Build history of the part. All positions in model axes, mm. A direction names the side the tool comes from. Give positions to 0.01 mm unless a question says otherwise; leave off trailing zeros. Write each loop counter-clockwise with the first axis right and the second up, starting at its lowest first coordinate (ties: lowest second). Pieces come first, ordered by that corner, then holes. Notation, with made-up numbers: (53.5, 31.25) -> (59.5, 31.25) arc R6 ccw to (59.5, 38.25) -> close; hole circle Ø5 at (-24, 19.5). An arc over 180 degrees is marked (long way). Write item = value, one per line. Start each with the question number.
Q1. Saw through at B-B, the plane y = 11. List the corners of the cut face in (x, z).
Q2. Drop flat-ended pins along their axis: P1, Ø3.5, axis at x = 8.5, z = -33, coming from the +Y side; P2, Ø8, axis at y = 14.5, z = 23.5, coming from the -X side; P3, Ø2.5, axis at x = 2.5, y = 2, coming from the +Z side. Give the stop position or say it passes through.
Q3. Saw through at D-D, the plane x = -16. List the corners of the cut face in (y, z), then the cut area to 3 significant figures.
Q4. Wall check: line 1 (Z direction, x = 33.5, y = 1.2); line 2 (Z direction, x = -30.5, y = 1.1); line 3 (Z direction, x = -2, y = 9.5). Give the ranges that are in metal, low to high.
Q5. Saw through at C-C, the plane z = 24. List the corners of the cut face in (x, y), then the cut area to 3 significant figures.
Q6. Saw through at A-A, the plane x = 23.5. List the corners of the cut face in (y, z).
Q7. Mould opens along X. For faces 4 (the face through (-37.5, 10, -19)), 5 (the face through (24, 20, 7.5)), 6 (the face through (1, 3, 0)), 7 (the face through (23.175, 32.536, 12.91)) say: pulls with the +X half, pulls with the -X half, needs draft (parallel to the pull), parting line crosses it, or undercut.
Q8. Tool access for faces 1 (the face through (24, 36, 18.171)), 2 (the face through (-9, 1, 31)), 3 (the face through (34.5, 12, -26)): list every direction of +Z, -Z, +X, -X, +Y, -Y with a clear straight run to the whole face (end or side of a thin tool).
Autodesk Inventor part; units mm, degrees
ref_plane "YZ Plane" through (0, 0, 0) normal (1, 0, 0) x (0, 1, 0)
ref_plane "XZ Plane" through (0, 0, 0) normal (0, 1, 0) x (-1, 0, 0)
ref_plane "XY Plane" through (0, 0, 0) normal (0, 0, 1) x (1, 0, 0)
sketch "Sketch1" plane through (0, 0, 0) normal (0, 1, 0) x (-1, 0, 0)
  line L0 (37.5, -31) -> (-37.5, -31)
  line L1 (-37.5, -31) -> (-37.5, 31)
  line L2 (-37.5, 31) -> (37.5, 31)
  line L3 (37.5, 31) -> (37.5, -31)
  line L4 (37.5, -31) -> (-37.5, 31) construction
  line L5 (-37.5, -31) -> (37.5, 31) construction
  point P0 (0, 0)
  dimension "d0" = 75
  dimension "d1" = 62
extrude "Extrusion1" add sketch "Sketch1" along normal blind 3
sketch "Sketch2" plane through (0, 3, 0) normal (0, 1, 0) x (1, 0, 0)
  line L0 (37.5, 31) -> (-37.5, 31)
  line L1 (-37.5, 31) -> (-37.5, -31)
  circle A0 centre (-30.5, -7.5) radius 2.5
  circle A1 centre (-30.5, -20) radius 2.5
  circle A2 centre (-16, 1) radius 2.5
  line L2 (-37.5, -31) -> (37.5, -31)
  line L3 (37.5, -31) -> (37.5, 31)
  line L4 (-30.5, -7.5) -> (-30.5, -31)
  point P0 (0, 0)
  dimension "d4" = 5
  dimension "d5" = 5
  dimension "d6" = 12.5
  dimension "d7" = 7
  dimension "d8" = 5
  dimension "d9" = 8.5
  dimension "d10" = 14.5
  dimension "d11" = 30
extrude "Extrusion2" cut sketch "Sketch2" against normal through all contours A0 | A1 L4 | L4 A1 | A2
sketch "Sketch3" plane through (0, 3, 0) normal (0, 1, 0) x (1, 0, 0)
  line L0 (-37.5, 31) -> (-37.5, -31)
  line L1 (37.5, -31) -> (37.5, 31)
  line L2 (-37.5, -20) -> (37.5, -20)
  line L3 (19.5, -32.5) -> (27.5, -32.5)
  line L4 (27.5, -32.5) -> (27.5, -7.5)
  line L5 (27.5, -7.5) -> (19.5, -7.5)
  line L6 (19.5, -7.5) -> (19.5, -32.5)
  line L7 (19.5, -32.5) -> (27.5, -7.5) construction
  line L8 (27.5, -32.5) -> (19.5, -7.5) construction
  circle A0 centre (-30.5, -20) radius 2.5
  point P0 (0, 0)
  point P1 (23.5, -20)
  dimension "d16" = 8
  dimension "d21" = 25
  dimension "d22" = 0
  dimension "d74" = 50
extrude "Extrusion3" add sketch "Sketch3" along normal blind 35 contours L6 L5 L4 L2 | L2 L4 L3 L6
sketch "Sketch4" plane through (27.5, 3, 32.5) normal (1, 0, 0) x (0, 0, -1)
  line L0 (25, 0) -> (1.5, 0)
  circle A0 centre (12.5, 18.5) radius 9
  line L1 (0, 35) -> (25, 35)
  line L2 (10.6712, 35) -> (14.3288, 35)
  line L3 (14.3288, 35) -> (14.3288, 27.3122)
  line L4 (14.3288, 27.3122) -> (10.6712, 27.3122)
  line L5 (10.6712, 27.3122) -> (10.6712, 35)
  line L6 (12.5, 35) -> (12.5, 0)
  line L7 (16.7228, 27.2139) -> (8.2773, 27.2139)
  line L8 (8.2773, 27.2139) -> (8.2773, 30.5)
  line L9 (8.2773, 30.5) -> (16.7228, 30.5)
  line L10 (16.7228, 30.5) -> (16.7228, 27.2139)
  line L11 (16.7228, 27.2139) -> (8.2773, 30.5) construction
  line L12 (8.2773, 27.2139) -> (16.7228, 30.5) construction
  point P0 (0, 0)
  point P1 (32.5, -3)
  point P2 (12.5, 28.8569)
  dimension "d86" = 18
  dimension "d87" = 18.5
  dimension "d88" = 3.6576
  dimension "d89" = 8.4455
  dimension "d90" = 3.2861
  dimension "d91" = 4.5
extrude "Extrusion4" cut sketch "Sketch4" against normal up to surface (8 mm away) contours A0 L6 L7 | L7 L6 L4 A0 | A0 L7 L6 | L4 L6 A0 | A0 L6 L9 L3 | L7 A0 L4 L6 | L6 L4 A0 | A0 L5 L9 L6 | L9 L6 L1 L3 | L9 L5 L1 L6
sketch "Sketch10" plane through (19.5, 3, 32.5) normal (0, 0, 1) x (1, 0, 0)
  circle A0 centre (4, 31) radius 1.5
  point P0 (6, -5)
  dimension "d49" = 3
sketch "Sketch9" plane through (19.5, 3, 32.5) normal (0, 0, 1) x (1, 0, 0)
  circle A0 centre (4, 31) radius 2
  point P0 (6, -5)
  dimension "d48" = 4
extrude "Extrusion9" cut sketch "Sketch10" against normal through all
extrude "Extrusion10" cut sketch "Sketch9" against normal up to surface (14.3288 mm away)
sketch "Sketch13" plane through (37.5, 0, -31) normal (0, 0, -1) x (-1, 0, 0)
  line L0 (75, 0) -> (75, 3)
  line L1 (0, 0) -> (75, 0)
  line L2 (75, 0) -> (75, 35)
  line L3 (75, 35) -> (0, 35)
  line L4 (0, 35) -> (0, 0)
  point P0 (37.5, 0)
  dimension "d71" = 35
extrude "Extrusion13" add sketch "Sketch13" along normal blind 3
sketch "Sketch14" plane through (0, 0, 0) normal (0, -1, 0) x (1, 0, 0)
  circle A0 centre (21, 27) radius 1.65
  circle A1 centre (33.5, 27) radius 1.65
  line L0 (33.5, 27) -> (21, 27)
  line L1 (21, 27) -> (21, -6)
  line L2 (21, -6) -> (33.5, -6)
  line L3 (33.5, -6) -> (33.5, 27)
  circle A2 centre (21, -6) radius 1.65
  circle A3 centre (33.5, -6) radius 1.65
  line L4 (37.5, -34) -> (37.5, 31)
  point P0 (0, 0)
  point P1 (37.5, -31)
  dimension "d75" = 12.5
  dimension "d76" = 3.3
  dimension "d77" = 3.3
  dimension "d78" = 3.3
  dimension "d79" = 3.3
  dimension "d81" = 33
  dimension "d82" = 25
  dimension "d93" = 4
extrude "Extrusion14" cut sketch "Sketch14" against normal up to next contours L0 L3 A1 | A1 L3 L0 | A3 L2 L3 | L3 L2 A3
sketch "Sketch15" plane through (37.5, 0, 31) normal (1, 0, 0) x (0, 0, -1)
  line L0 (62, 35) -> (62, 3)
  line L1 (0, 3) -> (62, 3)
  line L2 (62, 35) -> (44, 3)
  point P0 (31, 0)
  dimension "d94" = 18
extrude "Extrusion15" add sketch "Sketch15" against normal blind 3
sketch "Sketch16" plane through (-37.5, 0, 31) normal (-1, 0, 0) x (0, 0, 1)
  line L0 (-62, 3) -> (0, 3)
  line L1 (-62, 3) -> (-62, 35)
  line L2 (-62, 35) -> (-44, 3)
  point P0 (-31, 0)
  dimension "d97" = 18
extrude "Extrusion16" add sketch "Sketch16" against normal blind 3
sketch "Sketch17" plane through (0, 3, 0) normal (0, -1, 0) x (1, 0, 0)
  line L0 (19.5, 31) -> (27.5, 31)
  line L1 (27.5, 32.5) -> (27.5, 31)
  line L2 (19.5, 32.5) -> (27.5, 32.5)
  line L3 (19.5, 31) -> (19.5, 32.5)
  point P0 (0, 0)
extrude "Extrusion17" add sketch "Sketch17" along normal up to surface (3 mm away)
equation "\"d88\" = tslot_screw_width"
equation "\"d89\" = tslot_nut_width"
equation "\"d90\" = tslot_nut_thickness"
equation "\"Acrylic_thickness\" = 3.175"
equation "\"Wood_thickness\" = 5"
equation "\"Acrylic_kerf\" = 0"
equation "\"Wood_kerf\" = 0"
equation "\"resevoir_thickness\" = 12.7"
equation "\"acrylic_height\" = 304.8"
equation "\"acrylic_stopper\" = 125"
equation "\"arm_width\" = 25.4"
equation "\"arm_thickness\" = 1.5875"
equation "\"arm_length\" = 224.5"
equation "\"ball_joint_from_arm\" = 14.5"
equation "\"z_railA_from_screw\" = 35"
equation "\"z_railB_from_screw\" = 35"
equation "\"z_rail_D\" = 8"
equation "\"z_rail_support_hole\" = 5"
equation "\"z_screw_D\" = 8"
equation "\"lmk8uu_hole_space\" = 17"
equation "\"lmk8uu_hole_D\" = 3.3"
equation "\"lmk8uu_OD\" = 15"
equation "\"camera_arm_screw\" = 6.35"
equation "\"carrier_thickness\" = 5"
equation "\"turntable_ID\" = 145"
equation "\"turntable_outside_hole_radius\" = 92.72"
equation "\"turntable_inside_hole_radius\" = 79.16"
equation "\"turntable_hole_D\" = 5.6"
equation "\"oring_ID\" = 19.05"
equation "\"oring_OD\" = 23.8125"
equation "\"drive_set_screw\" = 2.5"
equation "\"drive_set_nut\" = 5"
equation "\"nema17_hole_D\" = 3.3"
equation "\"nema17_hole_space\" = 31"
equation "\"box_lid_from_back\" = 147.5"
equation "\"box_lid_slot_length\" = 0"
equation "\"mirror_thickness\" = 8"
equation "\"laser_angle\" = 25deg"
equation "\"laser_distance\" = 155.47675"
equation "\"m8_rail_height\" = 304.8"
equation "\"print_bed_drill\" = 7.9375"
equation "\"front_frame_inset\" = 28.04"
equation "\"petri_OD\" = 152.4"
equation "\"tslot_screw_length\" = 12.7"
equation "\"tslot_screw_width\" = 3.6576"
equation "\"tslot_nut_width\" = 8.4455"
equation "\"tslot_nut_thickness\" = 3.28612"
equation "\"center_frame_inset\" = 186.36"
equation "\"printer_z\" = 289"
equation "\"frame_tilt\" = 1deg"
equation "\"z_min_from_center\" = 72.6"
equation "\"crane_z\" = 25"
equation "\"tape_thickness\" = 2"
equation "\"tape_keep_out\" = 2"
equation "\"brass_keep_out\" = 8"
equation "\"crane_x\" = 245.2"
equation "\"brass_insert_drill\" = 4"
equation "\"bed_clamp_border\" = 15"
equation "\"tray_boarder\" = 15"
equation "\"motor_spacing\" = 296"
equation "\"threaded_rod_z\" = 203.2"
equation "\"linear_bearing_z\" = 304.8"
equation "\"clear_acrylic\" = 2"
equation "\"thin_acrylic\" = 3"
equation "\"carrier_z2\" = 283.6"
equation "\"carrier_z\" = 258.6"
equation "\"thick_acrylic\" = 5.6"
equation "\"linear_bearing_spacing\" = 216"
equation "\"laser_body_diameter\" = 12"
equation "\"stepper_body_diameter\" = 28"
equation "\"stepper_shaft_diameter\" = 5"
equation "\"m3_diameter\" = 3.15"
equation "\"stepper_screw_space\" = 35"
equation "\"m5_diameter\" = 5.25"
equation "\"subframe_y_offset\" = 27.5"
equation "\"laser_y_offset\" = 18.5"
equation "\"laser_diameter\" = 12"
equation "\"laser_y\" = 35"
equation "\"laser_z\" = 18"
properties part number "galvo holder" material "ABS Plastic"
Report:
q1.outline = (-37.5, -34) -> (37.5, -34) -> (37.5, -17.5) -> (34.5, -17.5) -> (34.5, -31) -> (-34.5, -31) -> (-34.5, -17.5) -> (-37.5, -17.5) -> close; (19.5, 7.5) -> (27.5, 7.5) -> (27.5, 32.5) -> (19.5, 32.5) -> close
q2.P1 = 35
q2.P2 = 19.5
q2.P3 = 31
q3.outline = (0, -34) -> (35, -34) -> (35, -31) -> (3, -31) -> (3, -3.5) -> (0, -3.5) -> close; (0, 1.5) -> (3, 1.5) -> (3, 31) -> (0, 31) -> close
q3.area = 276 mm2
q4.line_1 = -34 to -7.65, -4.35 to 25.35, 28.65 to 31
q4.line_2 = -34 to 5, 10 to 17.5, 22.5 to 31
q4.line_3 = -34 to -31
q5.outline = (-37.5, 0) -> (37.5, 0) -> (37.5, 3) -> (27.5, 3) -> (27.5, 13.44) -> (19.5, 13.44) -> (19.5, 3) -> (-37.5, 3) -> close; (19.5, 29.56) -> (27.5, 29.56) -> (27.5, 38) -> (19.5, 38) -> close; hole circle Ø4 at (23.5, 34)
q5.area = 363 mm2
q6.outline = (0, -34) -> (35, -34) -> (35, -31) -> (3, -31) -> (3, 7.5) -> (32.5, 7.5) -> (32.5, 18.17) -> (30.31, 18.17) arc R9 cw (long way) to (30.31, 21.83) -> (32, 21.83) -> (32, 32.5) -> (0, 32.5) -> close; (35.5, 7.5) -> (38, 7.5) -> (38, 18.17) -> (35.5, 18.17) -> close; (36, 21.83) -> (38, 21.83) -> (38, 32.5) -> (36, 32.5) -> close
q7.face_4 = pulls with the -X half
q7.face_5 = needs draft
q7.face_6 = undercut
q7.face_7 = undercut
q8.face_1 = +X, -X, +Y
q8.face_2 = +Z, -X, +Y, -Y
q8.face_3 = +Z, +Y
